Model file for the job. Use its own axes, mm. A direction names the side the tool comes from. Coordinates: 2 decimals unless noted, no trailing zeros. Order: outer loops, then holes, each group sorted by start corner. A loop starts at its lowest first (then second) coordinate and runs counter-clockwise, first axis right, second up.
Autodesk Fusion 360 part; units mm, degrees
sketch "Sketch1" plane through (0, 0, 0) normal (0, 0, 1) x (1, 0, 0)
  line L0 (0, 0) -> (140, 0)
  line L1 (140, 0) -> (140, 140)
  line L2 (140, 140) -> (0, 140)
  line L3 (0, 140) -> (0, 0)
  dimension "d1" = 140
  dimension "d2" = 140
extrude "Extrude1" add sketch "Sketch1" along normal blind 40
sketch "Sketch2" plane through (0, 0, 40) normal (0, 0, 1) x (-1, 0, 0)
  line L0 (0, -140) -> (0, 0)
  line L1 (0, 0) -> (-140, 0)
  line L2 (-140, 0) -> (-140, -140)
  line L3 (-140, -140) -> (0, -140)
  line L4 (0, 0) -> (-3, 0)
  line L5 (-3, 0) -> (-3, -3)
  line L6 (-3, -3) -> (0, -3)
  line L7 (0, -3) -> (0, 0)
  line L8 (-140, -140) -> (-137, -140)
  line L9 (-137, -140) -> (-137, -137)
  line L10 (-137, -137) -> (-140, -137)
  line L11 (-140, -137) -> (-140, -140)
  line L12 (-3, -3) -> (-137, -3)
  line L13 (-137, -3) -> (-137, -137)
  line L14 (-137, -137) -> (-3, -137)
  line L15 (-3, -137) -> (-3, -3)
  dimension "d5" = 3
  dimension "d6" = 3
  dimension "d7" = 3
  dimension "d8" = 3
extrude "Extrude6" cut sketch "Sketch2" against normal blind 27 contours L12 L13 L14 L15
sketch "Sketch5" plane through (0, 0, 0) normal (0, -1, 0) x (1, 0, 0)
  line L0 (0, 0) -> (140, 0)
  line L1 (140, 0) -> (140, 40)
  line L2 (140, 40) -> (0, 40)
  line L3 (0, 40) -> (0, 0)
  line L4 (10, 40) -> (25, 25)
  line L5 (25, 25) -> (115, 25)
  line L6 (115, 25) -> (130, 40)
extrude "Extrude7" cut sketch "Sketch5" against normal blind 5 contours L2 L4 L5 L6
Q1. Probe line 1 (X direction, y = 6, z = 15); line 2 (Y direction, x = 43.5, z = 30). List the from-to ranges inside material, lowest first.
Established:
line 1: x = 0 to 3, 137 to 140
line 2: y = 137 to 140
Q2. Cut at D-D, the plane z = 16.5. List the corners of the cut face in (x, y), plus the area to 3 significant figures.
Established:
outline: (0, 0) - (140, 0) - (140, 140) - (0, 140) - close; hole (3, 3) - (137, 3) - (137, 137) - (3, 137) - close
area: 1,640 mm2
Q3. Drop flat-ended pins along their axis: P1, Ø0.9, axis at x = 47.5, y = 1, coming from the +Z side; P2, Ø10, axis at x = 41.5, y = 77.5, coming from the +Z side. Give the stop position or say it passes through.
Established:
P1: stops at z = 25
P2: stops at z = 13
Q4. Which spindle directions (+Z, -Z, +X, -X, +Y, -Y) get a long thin tool onto all of the face, cutting with end or side? Do faces 4 (the face through (69, 3, 21)), 5 (the face through (122, 1, 32)), 6 (the face through (70, 138, 40)). Say none if no direction does.
Established:
face 4: +Z
face 5: +Z, -Y
face 6: +Z, +X, -X, +Y, -Y
Q5. Cut at A-A, the plane x = 103. List the corners of the cut face in (y, z).
Established:
outline: (0, 0) - (140, 0) - (140, 40) - (137, 40) - (137, 13) - (3, 13) - (3, 25) - (0, 25) - close
Q6. Mould opens along Y. For faces 1 (the face through (71, 69, 13)), 2 (the face through (17, 1, 33)), 3 (the face through (71, 140, 20)) say: pulls with the +Y half, pulls with the -Y half, needs draft (parallel to the pull), parting line crosses it, or undercut.
Established:
face 1: undercut
face 2: needs draft
face 3: pulls with the +Y half
Q7. Cut at B-B, the plane z = 37. List the corners of the cut face in (x, y).
Established:
outline: (0, 0) - (13, 0) - (13, 3) - (3, 3) - (3, 137) - (137, 137) - (137, 3) - (127, 3) - (127, 0) - (140, 0) - (140, 140) - (0, 140) - close
Q8. Cut at C-C, the plane y = 77.5. List the corners of the cut face in (x, z).
Established:
outline: (0, 0) - (140, 0) - (140, 40) - (137, 40) - (137, 13) - (3, 13) - (3, 40) - (0, 40) - close
